Autodesk Inventor part; units mm, degrees
ref_plane "작업 평면1" through (0, 0, -43.75) normal (0, 0, 1) x (1, 0, 0)
ref_plane "YZ Plane" through (0, 0, 0) normal (1, 0, 0) x (0, 1, 0)
ref_plane "XZ Plane" through (0, 0, 0) normal (0, 1, 0) x (-1, 0, 0)
sketch "스케치1" plane through (0, 0, 0) normal (0, 0, 1) x (1, 0, 0)
  line L0 (-7.5, -15) -> (7.5, -15)
  line L1 (7.5, -15) -> (7.5, 15)
  line L2 (7.5, 15) -> (-7.5, 15)
  line L3 (-7.5, 15) -> (-7.5, -15)
  point P0 (0, 0)
  dimension "d0" = 15
  dimension "d1" = 30
  dimension "d2" = 15
  dimension "d3" = 7.5
extrude "돌출1" add sketch "스케치1" against normal blind 37.5
sketch "스케치2" plane through (0, 0, -37.5) normal (0, 0, -1) x (-1, 0, 0)
  line L0 (5, 11.25) -> (-5, 11.25)
  line L1 (-5, 11.25) -> (-5, -11.25)
  line L2 (-5, -11.25) -> (5, -11.25)
  line L3 (5, -11.25) -> (5, 11.25)
  line L4 (5, 11.25) -> (-5, -11.25) construction
  line L5 (-5, 11.25) -> (5, -11.25) construction
  line L6 (-4, -10) -> (4, -10)
  line L7 (4, -10) -> (4, 10)
  line L8 (4, 10) -> (-4, 10)
  line L9 (-4, 10) -> (-4, -10)
  line L10 (-4, -10) -> (4, 10) construction
  line L11 (4, -10) -> (-4, 10) construction
  point P0 (0, 0)
  dimension "d6" = 10
  dimension "d7" = 22.5
  dimension "d10" = 8
  dimension "d11" = 20
extrude "돌출2" add sketch "스케치2" along normal blind 50
sketch "스케치3" plane through (0, 0, 0) normal (0, 0, 1) x (1, 0, 0)
  line L0 (-3.95, -5) -> (3.95, -5)
  line L1 (3.95, -5) -> (3.95, 5)
  line L2 (3.95, 5) -> (-3.95, 5)
  line L3 (-3.95, 5) -> (-3.95, -5)
  line L4 (-3.95, -5) -> (3.95, 5) construction
  line L5 (3.95, -5) -> (-3.95, 5) construction
  point P0 (0, 0)
  dimension "d12" = 7.9
  dimension "d13" = 10
extrude "돌출3" add sketch "스케치3" along normal blind 15
sketch "스케치4" plane through (3.95, -5, 0) normal (1, 0, 0) x (0, 0, -1)
  circle A0 centre (-10, 5) radius 2.1
  line L0 (0, 0) -> (-15, 0)
  line L1 (-15, 0) -> (-15, 10)
  point P0 (0, 5)
  dimension "d16" = 4.2
  dimension "d17" = 5
  dimension "d18" = 5
extrude "돌출4" cut sketch "스케치4" against normal blind 15
sketch "스케치5" plane through (0, 0, -87.5) normal (0, 0, -1) x (-1, 0, 0)
  line L0 (-5, 11.25) -> (5, 11.25)
  line L1 (5, -11.25) -> (-5, -11.25)
  line L2 (5, 11.25) -> (-5, 11.25)
  line L3 (-5, 11.25) -> (-5, -11.25)
  line L4 (-5, -11.25) -> (5, -11.25)
  line L5 (5, -11.25) -> (5, 11.25)
  point P0 (7.5, 15)
  point P1 (-7.5, -15)
extrude "돌출5" add sketch "스케치5" against normal blind 2
ref_plane "작업 평면1" through (0, 0, -43.75) normal (0, 0, 1) x (1, 0, 0)
mirror "미러1" about plane through (0, 0, -43.75) normal (0, 0, 1) of "돌출3"
mirror "미러2" about plane through (0, 0, -43.75) normal (0, 0, 1) of "돌출4"
fillet "모깎기1" radius 4 4 edges at (0, -5, 15) (0, 5, 15) (0, -5, -102.5) (0, 5, -102.5)
properties part number "각도조절 액추에이터_최소" material "납"
The listing builds one solid part. Answer for the finished solid, in the listing's coordinates (mm). A direction names the side the tool comes from. Round coordinates to 2 decimals unless told otherwise and drop trailing zeros. Order: outer loops, then holes, each group sorted by start corner. A loop starts at its lowest first (then second) coordinate and runs counter-clockwise, first axis right, second up. Notation, with made-up numbers: M 38,-32.75 L 52,-32.75 A25 ccw 52,-5.75 Z; hole C 72,51.25 d9. An arc over 180 degrees is marked long. Answer in a Markdown table with one row per item. Add a question column.
1) Flat-ended cylindrical pins translate along their axes: pin 1 Ø8.5 at (x, z) = (1, -95) entering from -Y; pin 2 Ø4 at (x, z) = (1, -71.5) entering from +Y; pin 3 Ø10 at (y, z) = (3.5, -54.5) entering from -X. Find the tip coordinate at first contact, or state that the pin passes through.
2) The part is cut by section B-B on y = -8.75. Determine the outline of the cut face in (x, z).
3) Which of the six approach directions +Z, -Z, +X, -X, +Y, -Y give full straight-line access (tool end or side, diameter ignored) to faces 1 (the face through (0, 5, -93)), 2 (the face through (0, -11.25, -62)), 3 (the face through (0, -10, -61))?
4) Consider line 1 along X through (y, z) = (-7.5, -38); line 2 along Y through (x, z) = (-1.5, -97.5); line 3 along Z through (x, y) = (2.5, -5.5). Determine where each line is inside the solid, lowest interval first. Write a range as from..to.
5) The part is cut by section C-C on x = -1.5. Determine the outline of the cut face in (y, z), plus the area to 3 significant figures.
6) Determine the mould class of faces 4 (the face through (0, 5, 5)), 5 (the face through (-5, 0, 0)), 6 (the face through (0, 0, -37.5)) for opening direction Y: pulls with the +Y half, pulls with the -Y half, needs draft (parallel to the pull), parting line crosses it, or undercut.
7) The part is cut by section D-D on y = 0. Determine the outline of the cut face in (x, z), plus the area to 3 significant figures.
8) The part is cut by section A-A on z = -97.5. Determine the outline of the cut face in (x, y), plus the area to 3 significant figures.
Findings below:
| question | item | result |
|---|---|---|
| 1 | pin 1 | stops at y = -5 |
| 1 | pin 2 | stops at y = 11.25 |
| 1 | pin 3 | stops at x = -5 |
| 2 | outline | M -7.5,-37.5 L -5,-37.5 L -5,-87.5 L 5,-87.5 L 5,-37.5 L 7.5,-37.5 L 7.5,0 L -7.5,0 Z; hole M -4,-85.5 L 4,-85.5 L 4,-37.5 L -4,-37.5 Z |
| 3 | face 1 | -Z, +X, -X, +Y |
| 3 | face 2 | -Z, +X, -X, -Y |
| 3 | face 3 | none |
| 4 | line 1 | x = -5..-4, 4..5 |
| 4 | line 2 | y = -5..-2.1, 2.1..5 |
| 4 | line 3 | z = -87.5..-85.5, -37.5..0 |
| 5 | outline | M -15,-37.5 L -11.25,-37.5 L -11.25,-87.5 L -5,-87.5 L -5,-98.5 A4 ccw -1,-102.5 L 1,-102.5 A4 ccw 5,-98.5 L 5,-87.5 L 11.25,-87.5 L 11.25,-37.5 L 15,-37.5 L 15,0 L 5,0 L 5,11 A4 ccw 1,15 L -1,15 A4 ccw -5,11 L -5,0 L -15,0 Z; hole M -10,-85.5 L 10,-85.5 L 10,-37.5 L -10,-37.5 Z; hole C 0,-97.5 d4.2; hole C 0,10 d4.2 |
| 5 | area | 1,550 mm² |
| 6 | face 4 | pulls with the +Y half |
| 6 | face 5 | needs draft |
| 6 | face 6 | undercut |
| 7 | outline | M -7.5,-37.5 L -5,-37.5 L -5,-87.5 L -3.95,-87.5 L -3.95,-95.4 L 3.95,-95.4 L 3.95,-87.5 L 5,-87.5 L 5,-37.5 L 7.5,-37.5 L 7.5,0 L 3.95,0 L 3.95,7.9 L -3.95,7.9 L -3.95,0 L -7.5,0 Z; M -3.95,-102.5 L 3.95,-102.5 L 3.95,-99.6 L -3.95,-99.6 Z; M -3.95,12.1 L 3.95,12.1 L 3.95,15 L -3.95,15 Z; hole M -4,-85.5 L 4,-85.5 L 4,-37.5 L -4,-37.5 Z |
| 7 | area | 849 mm² |
| 8 | outline | M -3.95,-5 L 3.95,-5 L 3.95,-2.1 L -3.95,-2.1 Z; M -3.95,2.1 L 3.95,2.1 L 3.95,5 L -3.95,5 Z |
| 8 | area | 45.8 mm² |
